Work out the finished part from the listing and answer in its coordinate system (mm). A direction names the side the tool comes from. Give positions to 0.01 mm unless a question says otherwise; leave off trailing zeros. Loops run counter-clockwise (first coordinate to the right, second up) from the corner with the lowest first, then second, coordinate; pieces in that order, holes last. Notation, with made-up numbers: (-25.5, 75) - (32.5, 75) arc R23 cw to (32.5, 110) - close; hole circle Ø7 at (26, -15.5). An arc over 180 degrees is marked (long way). One line per item, written item: value.
from build123d import *

# Parameters (mm, degrees)
BOSS_EXTRUDE1_DEPTH                                 = 5
CBORE_FOR_M8_HEX_SOCKET_HEAD_CAP_SCREW1_D           = 9
CBORE_FOR_M8_HEX_SOCKET_HEAD_CAP_SCREW1_CBORE_D     = 15
CBORE_FOR_M8_HEX_SOCKET_HEAD_CAP_SCREW1_CBORE_DEPTH = 8.6
SKETCH5_R                                           = 9.5
CUT_EXTRUDE2_DEPTH                                  = 8
SKETCH6_R                                           = 8
CUT_EXTRUDE3_DEPTH                                  = 465.530946224
FILLET1_R                                           = 25
M10_CLEARANCE_HOLE1_D                               = 11
M10_CLEARANCE_HOLE1_DEPTH                           = 25
M10_CLEARANCE_HOLE1_TIP                             = 3.304733405


with BuildPart() as part:
    # Sketch1 → Boss-Extrude1 (new, symmetric)
    with BuildSketch(Plane.XY):
        Polygon((-115, 450), (-115, 0), (115, 0), (115, 200), (-15, 450), align=None)
    extrude(amount=BOSS_EXTRUDE1_DEPTH, both=True)

    # CBORE for M8 Hex Socket Head Cap Screw1 (through all)
    with Locations(Plane.XY.offset(5)):
        with Locations((-90, 17.5), (-45, 17.5), (45, 17.5), (90, 17.5), (0, 17.5), (-90, 62.5), (-45, 62.5), (45, 62.5), (90, 62.5), (0, 62.5)):
            CounterBoreHole(CBORE_FOR_M8_HEX_SOCKET_HEAD_CAP_SCREW1_D / 2, CBORE_FOR_M8_HEX_SOCKET_HEAD_CAP_SCREW1_CBORE_D / 2, CBORE_FOR_M8_HEX_SOCKET_HEAD_CAP_SCREW1_CBORE_DEPTH)

    # Sketch5 → Cut-Extrude2 (cut)
    with BuildSketch(Plane.XY.offset(5)):
        with Locations((-93.85, 428.85)):
            Circle(SKETCH5_R)
    extrude(amount=-CUT_EXTRUDE2_DEPTH, mode=Mode.SUBTRACT)

    # Sketch6 → Cut-Extrude3 (cut, through all)
    with BuildSketch(Plane.XY.offset(-3)):
        with Locations((-93.85, 428.85)):
            Circle(SKETCH6_R)
    extrude(amount=-CUT_EXTRUDE3_DEPTH, mode=Mode.SUBTRACT)

    # Fillet1
    fillet1_edges = [part.edges().sort_by_distance(p)[0] for p in [
        (-15, 450, 0),
        (115, 200, 0),
    ]]
    fillet(fillet1_edges, radius=FILLET1_R)

    # M10 Clearance Hole1
    with Locations(Plane.XY.offset(5)):
        with Locations((-92.5, 387.5), (-92.5, 342.5)):
            Hole(M10_CLEARANCE_HOLE1_D / 2, depth=M10_CLEARANCE_HOLE1_DEPTH)
            with Locations((0, 0, -(M10_CLEARANCE_HOLE1_DEPTH + M10_CLEARANCE_HOLE1_TIP / 2))):  # 118° drill point
                Cone(0, M10_CLEARANCE_HOLE1_D / 2, M10_CLEARANCE_HOLE1_TIP, mode=Mode.SUBTRACT)


solid = part.part
1. Flat-ended cylindrical pins translate along their axes: pin 1 Ø11.5 at (x, y) = (-45, 62.5) entering from +Z; pin 2 Ø9 at (x, y) = (-92.5, 342.5) entering from -Z; pin 3 Ø1.5 at (x, z) = (74.5, -2.5) entering from +Y. Find the tip coordinate at first contact, or state that the pin passes through.
Output:
pin 1: stops at z = -3.6
pin 2: passes through
pin 3: stops at y = 279.33
2. For faces 1 (the cylindrical face through (94.496, 17.698, -4.31)), 2 (the cylindrical face through (-37.846, 19.753, 0.76)), determine the directions among +Z, -Z, +X, -X, +Y, -Y from which every point of the face is accessible in a straight line to the end or side of a thin tool.
Output:
face 1: +Z, -Z
face 2: +Z
3. Section D-D (y = 342.5) is taken. Write down the section's boundary in (x, z).
Output:
outline: (-115, -5) - (-98, -5) - (-98, 5) - (-115, 5) - close; (-87, -5) - (40.9, -5) - (40.9, 5) - (-87, 5) - close
4. Section C-C (x = 0) is taken. Write down the section's boundary in (y, z).
Output:
outline: (0, -5) - (13, -5) - (13, -3.6) - (10, -3.6) - (10, 5) - (0, 5) - close; (22, -5) - (58, -5) - (58, -3.6) - (55, -3.6) - (55, 5) - (25, 5) - (25, -3.6) - (22, -3.6) - close; (67, -5) - (421.15, -5) - (421.15, 5) - (70, 5) - (70, -3.6) - (67, -3.6) - close
5. Section B-B (z = 1) is taken. Count the separate pieces of the cut face and the enclosed holes in it, and give its area (3 significant figures).
Output:
separate pieces: 1
enclosed holes: 13
area: 85,000 mm²
6. The mould has two halves that part along X. Classify faces 3 (the flat face through (-27, 178, -5)), 4 (the flat face through (52.933, 319.36, 0.07)), 5 (the flat face through (-98.12, 421.86, -3)): released by +X, released by -X, zero draft, split by the parting line, or undercut.
Output:
face 3: zero draft
face 4: released by +X
face 5: undercut
7. Section A-A (y = 387.5) is taken. Write down the section's boundary in (x, z).
Output:
outline: (-115, -5) - (-98, -5) - (-98, 5) - (-115, 5) - close; (-87, -5) - (17.5, -5) - (17.5, 5) - (-87, 5) - close
8. Find the intervals of material crossed by line 1 along Y through (x, z) = (-4, -3.5); line 2 along Y through (x, z) = (0, -4); line 3 along Y through (x, z) = (-90, -4.05), in increasing order.
Output:
line 1: y = 0 to 11.16, 23.84 to 56.16, 68.84 to 428.85
line 2: y = 0 to 13, 22 to 58, 67 to 421.15
line 3: y = 0 to 13, 22 to 58, 67 to 337.6, 347.4 to 382.6, 392.4 to 421.84, 435.86 to 450
